Here's the drawing with two shaded views (mm, measured from the low corner). I have some questions. A direction names the side the tool comes from. Coordinates: 2 decimals unless noted, no trailing zeros. Write each loop counter-clockwise with the first axis right and the second up, starting at its lowest first coordinate (ties: lowest second). Pieces come first, ordered by that corner, then holes. Notation, with made-up numbers: (-3, 49) -> (3, 49) arc R11 cw to (3, 56) -> close; hole circle Ø8 at (66.25, 53.5). An arc over 180 degrees is marked (long way). Put each result on its own line as item: value.
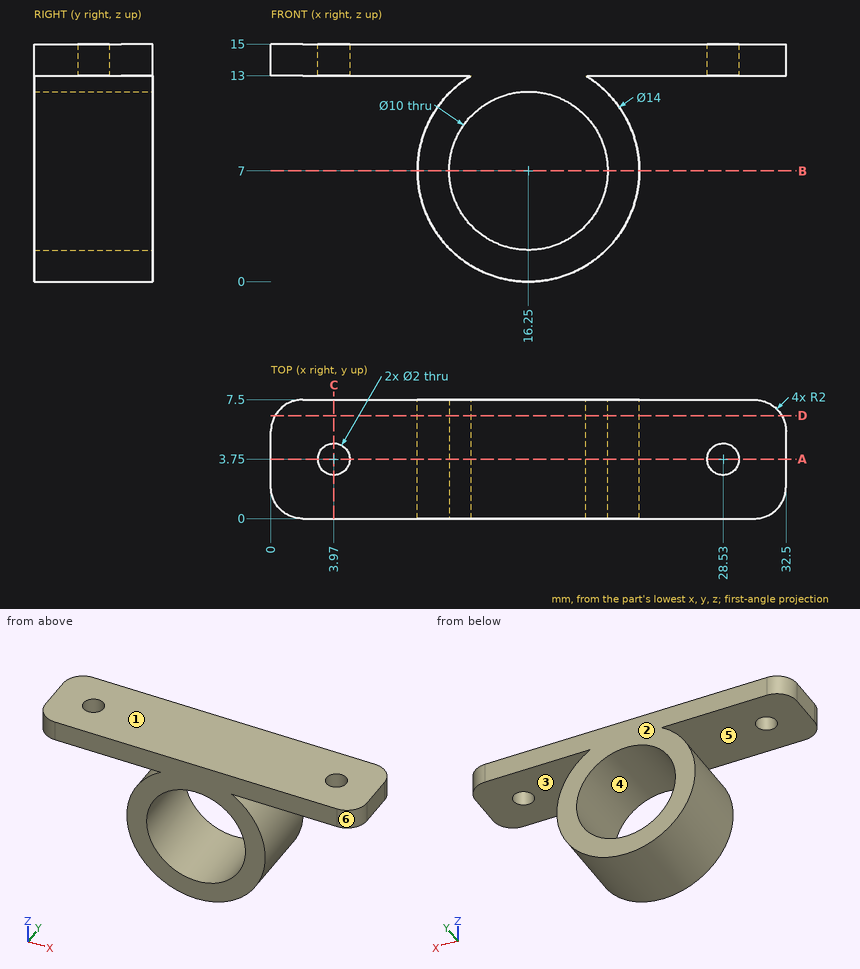
Item 1: For P1, Ø3, axis at x = 3.97, y = 3.75, coming from the -Z side; P2, Ø6, axis at x = 6, z = 2, coming from the -Y side; P3, Ø4, axis at y = 2.5, z = 8.5, coming from the -X side; P4, Ø1, axis at y = 1, z = 3, coming from the -X side, each with a flat end and sliding along its axis, tell me the tip position at first contact or that it passes through.
Output:
P1: stops at z = 13
P2: passes through
P3: stops at x = 9.25
P4: stops at x = 10.19
Item 2: Imagine slicing it at C-C on x = 3.97. Write out the boundary of the cut face in (y, z).
Output:
outline: (0, 13) -> (2.75, 13) -> (2.75, 15) -> (0, 15) -> close; (4.75, 13) -> (7.5, 13) -> (7.5, 15) -> (4.75, 15) -> close
Item 3: Imagine slicing it at B-B on z = 7. Write out the boundary of the cut face in (x, y), then the cut area to 3 significant figures.
Output:
outline: (9.25, 0) -> (11.25, 0) -> (11.25, 7.5) -> (9.25, 7.5) -> close; (21.25, 0) -> (23.25, 0) -> (23.25, 7.5) -> (21.25, 7.5) -> close
area: 30.0 mm²
Item 4: Imagine slicing it at A-A on y = 3.75. Write out the boundary of the cut face in (x, z).
Output:
outline: (0, 13) -> (2.97, 13) -> (2.97, 15) -> (0, 15) -> close; (4.97, 13) -> (12.64, 13) arc R7 ccw (long way) to (19.86, 13) -> (27.53, 13) -> (27.53, 15) -> (4.97, 15) -> close; (29.53, 13) -> (32.5, 13) -> (32.5, 15) -> (29.53, 15) -> close; hole circle Ø10 at (16.25, 7)
Item 5: Which directions (+Z, -Z, +X, -X, +Y, -Y) give clear straight access to the entire face, cutting with the end or side of a thin tool? Please do the marked faces 5 and 6.
Output:
face 5: -X, +Y, -Y
face 6: +Z, -Z, +X, -Y
Item 6: Imagine slicing it at D-D on y = 6.5. Write out the boundary of the cut face in (x, z), then the cut area to 3 significant figures.
Output:
outline: (0.27, 13) -> (12.64, 13) arc R7 ccw (long way) to (19.86, 13) -> (32.23, 13) -> (32.23, 15) -> (0.27, 15) -> close; hole circle Ø10 at (16.25, 7)
area: 134 mm²
Item 7: If we mould it in two halves opening along Z, with no side actions, what happens to the marked faces 1, 2, 3 and 4? For each: released by +Z, released by -Z, zero draft, split by the parting line, or undercut.
Output:
face 1: released by +Z
face 2: zero draft
face 3: undercut
face 4: undercut
Item 8: Please list where these lines run through material, in increasing order: line 1 along X through (y, z) = (3.75, 6.75); line 2 along Z through (x, y) = (12, 3); line 3 along Z through (x, y) = (8, 0.5). Write a range as from..to.
Output:
line 1: x = 9.25..11.26, 21.24..23.25
line 2: z = 1.44..4.37, 9.63..12.56, 13..15
line 3: z = 13..15
